Geometry check sheet. Reference: the model listing, model coordinates, mm. A direction names the side the tool comes from. Coordinates: 2 decimals unless noted, no trailing zeros. Order: outer loops, then holes, each group sorted by start corner. A loop starts at its lowest first (then second) coordinate and runs counter-clockwise, first axis right, second up. Notation, with made-up numbers: (47.25, 32) - (68.25, 32) arc R26 ccw to (68.25, 55) - close; hole circle Ø6 at (-26.75, 24). An arc over 180 degrees is marked (long way). Put each result on its own line as item: value.
Autodesk Inventor part; units mm, degrees
ref_plane "YZ Plane" through (0, 0, 0) normal (1, 0, 0) x (0, 1, 0)
ref_plane "XZ Plane" through (0, 0, 0) normal (0, 1, 0) x (-1, 0, 0)
ref_plane "XY Plane" through (0, 0, 0) normal (0, 0, 1) x (1, 0, 0)
ref_plane "Work Plane1" through (0, 0, 0) normal (0, 0, 1) x (1, 0, 0)
sketch "Sketch1" plane through (0, 0, 0) normal (0, 0, 1) x (1, 0, 0)
  circle A0 centre (-18, 0) radius 2.45 construction
  circle A1 centre (-32.0354, 0) radius 2.45 construction
  circle A2 centre (-48, 0) radius 3.05 construction
  line L0 (18, 6) -> (-54, 6) construction
  line L1 (-54, -6) -> (-54, 6) construction
  line L2 (-54, -6) -> (18, -6) construction
  line L3 (18, -6) -> (18, 6) construction
  circle A3 centre (12, 0) radius 3.05 construction
  circle A4 centre (-3.9646, 0) radius 2.45 construction
  circle A5 centre (-18, -62.5107) radius 2.45 construction
  circle A6 centre (-3.9646, -62.1646) radius 2.45 construction
  circle A7 centre (12, -70) radius 3.05 construction
  line L4 (-32.0354, -67.7344) -> (-3.9646, -67.7344) construction
  line L5 (-3.9646, -67.7344) -> (14.2856, -76.6915) construction
  line L6 (14.2856, -76.6915) -> (18.6915, -67.7144) construction
  line L7 (18.6915, -67.7144) -> (-2.5545, -57.2869) construction
  line L8 (-33.4455, -57.2869) -> (-2.5545, -57.2869) construction
  line L9 (-54.6915, -67.7144) -> (-33.4455, -57.2869) construction
  line L10 (-50.2856, -76.6915) -> (-54.6915, -67.7144) construction
  line L11 (-32.0354, -67.7344) -> (-50.2856, -76.6915) construction
  circle A8 centre (-48, -70) radius 3.05 construction
  circle A9 centre (-32.0354, -62.1646) radius 2.45 construction
  line L12 (-30, -24.7225) -> (-6, -24.7225) construction
  line L13 (-6, -24.7225) -> (-6, -18.4525) construction
  line L14 (-6, -18.4525) -> (-30, -18.4525) construction
  line L15 (-30, -18.4525) -> (-30, -24.7225) construction
  line L16 (-6, -33.7225) -> (-11.7463, -33.7225) construction
  line L17 (-6, -33.34) -> (-6, -33.7225) construction
  line L18 (-6, -33.34) -> (-11.7042, -33.34) construction
  line L19 (-6, -32.95) -> (-6, -33.34) construction
  line L20 (-6, -32.95) -> (-11.6853, -32.95) construction
  line L21 (-6, -32.56) -> (-6, -32.95) construction
  line L22 (-6, -32.56) -> (-11.6906, -32.56) construction
  line L23 (-6, -32.17) -> (-6, -32.56) construction
  line L24 (-6, -32.17) -> (-11.72, -32.17) construction
  line L25 (-6, -31.78) -> (-6, -32.17) construction
  line L26 (-6, -31.78) -> (-11.7739, -31.78) construction
  line L27 (-6, -31.39) -> (-6, -31.78) construction
  line L28 (-6, -31.39) -> (-11.8531, -31.39) construction
  line L29 (-6, -31) -> (-6, -31.39) construction
  line L30 (-6, -31) -> (-11.9583, -31) construction
  line L31 (-6, -30.61) -> (-6, -31) construction
  line L32 (-6, -30.61) -> (-12.0912, -30.61) construction
  line L33 (-6, -30.22) -> (-6, -30.61) construction
  line L34 (-6, -30.22) -> (-12.2534, -30.22) construction
  line L35 (-6, -29.83) -> (-6, -30.22) construction
  line L36 (-6, -29.83) -> (-12.4478, -29.83) construction
  line L37 (-6, -29.44) -> (-6, -29.83) construction
  line L38 (-6, -29.44) -> (-12.6777, -29.44) construction
  line L39 (-6, -29.05) -> (-6, -29.44) construction
  line L40 (-6, -29.05) -> (-12.948, -29.05) construction
  line L41 (-6, -28.66) -> (-6, -29.05) construction
  line L42 (-6, -28.66) -> (-13.2656, -28.66) construction
  line L43 (-6, -24.7225) -> (-6, -28.66) construction
  line L44 (-30, -24.7225) -> (-6, -24.7225) construction
  line L45 (-30, -28.66) -> (-30, -24.7225) construction
  line L46 (-22.7344, -28.66) -> (-30, -28.66) construction
  line L47 (-30, -29.05) -> (-30, -28.66) construction
  line L48 (-23.052, -29.05) -> (-30, -29.05) construction
  line L49 (-30, -29.44) -> (-30, -29.05) construction
  line L50 (-23.3223, -29.44) -> (-30, -29.44) construction
  line L51 (-30, -29.83) -> (-30, -29.44) construction
  line L52 (-23.5522, -29.83) -> (-30, -29.83) construction
  line L53 (-30, -30.22) -> (-30, -29.83) construction
  line L54 (-23.7466, -30.22) -> (-30, -30.22) construction
  line L55 (-30, -30.61) -> (-30, -30.22) construction
  line L56 (-23.9088, -30.61) -> (-30, -30.61) construction
  line L57 (-30, -31) -> (-30, -30.61) construction
  line L58 (-24.0417, -31) -> (-30, -31) construction
  line L59 (-30, -31.39) -> (-30, -31) construction
  line L60 (-24.1469, -31.39) -> (-30, -31.39) construction
  line L61 (-30, -31.78) -> (-30, -31.39) construction
  line L62 (-24.2261, -31.78) -> (-30, -31.78) construction
  line L63 (-30, -32.17) -> (-30, -31.78) construction
  line L64 (-24.28, -32.17) -> (-30, -32.17) construction
  line L65 (-30, -32.56) -> (-30, -32.17) construction
  line L66 (-24.3094, -32.56) -> (-30, -32.56) construction
  line L67 (-30, -32.95) -> (-30, -32.56) construction
  line L68 (-24.3147, -32.95) -> (-30, -32.95) construction
  line L69 (-30, -33.34) -> (-30, -32.95) construction
  line L70 (-24.2958, -33.34) -> (-30, -33.34) construction
  line L71 (-30, -33.7225) -> (-30, -33.34) construction
  line L72 (-24.2537, -33.7225) -> (-30, -33.7225) construction
  line L73 (-7.4129, -57.0165) -> (-7.4129, -24.5897) construction
  line L74 (-21.9151, -37.7958) -> (-30, -37.7958) construction
  line L75 (-30, -37.7958) -> (-30, -44.4525) construction
  line L76 (-30, -44.4525) -> (-6, -44.4525) construction
  line L77 (-6, -44.4525) -> (-6, -37.7958) construction
  line L78 (-6, -37.7958) -> (-14.0849, -37.7958) construction
  line L79 (-29, -9.8284) -> (-29, -53.5585)
  line L80 (-7, -53.5585) -> (-7, -9.8284)
  line L81 (-7.4685, -54.8448) -> (-16.4685, -65.5601)
  line L82 (-19.5315, -65.5601) -> (-28.5315, -54.8448)
  line L83 (-6.4142, -8.4142) -> (2, 0)
  line L84 (-7, -9) -> (4.8995, -9) construction
  line L85 (2.5858, 1.4142) -> (2.5858, 4)
  line L86 (-29.5858, -8.4142) -> (-38, 0)
  line L87 (-29, -9) -> (-17.1005, -9) construction
  line L88 (-38.5858, 1.4142) -> (-38.5858, 4)
  line L89 (0.5858, 6) -> (-36.5858, 6)
  circle A10 centre (-3.9646, 0) radius 1.45
  circle A11 centre (-32.0354, 0) radius 1.45
  circle A12 centre (-18, -62.5107) radius 1.45
  arc A13 (-19.5315, -65.5601) -> (-16.4685, -65.5601) centre (-18, -64.2738) ccw
  arc A14 (-7.4685, -54.8448) -> (-7, -53.5585) centre (-9, -53.5585) ccw
  arc A15 (-29, -53.5585) -> (-28.5315, -54.8448) centre (-27, -53.5585) ccw
  arc A16 (-6.4142, -8.4142) -> (-7, -9.8284) centre (-5, -9.8284) ccw
  arc A17 (-29, -9.8284) -> (-29.5858, -8.4142) centre (-31, -9.8284) ccw
  arc A18 (-36.5858, 6) -> (-38.5858, 4) centre (-36.5858, 4) ccw
  arc A19 (2.5858, 4) -> (0.5858, 6) centre (0.5858, 4) ccw
  arc A20 (2, 0) -> (2.5858, 1.4142) centre (0.5858, 1.4142) ccw
  arc A21 (-38.5858, 1.4142) -> (-38, 0) centre (-36.5858, 1.4142) ccw
  arc A22 (-21.9151, -37.7958) -> (-14.0849, -37.7958) centre (-18, -32.8401) ccw
  arc A23 (-24.2537, -33.7225) -> (-11.7463, -33.7225) centre (-18, -32.8401) ccw
  point P0 (0, 0)
  point P1 (2.5858, 6)
  point P2 (-38.5858, 6)
  dimension "d0" = 1
  dimension "d1" = 1
  dimension "d4" = 45
  dimension "d5" = 135
  dimension "d6" = 2.9
  dimension "d7" = 2.9
  dimension "d8" = 2.9
  dimension "d9" = 2
extrude "Extrusion1" add sketch "Sketch1" along normal blind 4
sketch "Sketch2" plane through (-29, -53.5585, 0) normal (-1, 0, 0) x (0, 0, 1)
  line L0 (-1.5567, 7.7184) -> (-1.5567, 33.7184)
  line L1 (4.4433, 27.7184) -> (4.4433, 13.7184)
  line L2 (-41.5567, 33.7184) -> (-41.5567, 7.7184)
  line L3 (10.4433, 9.1059) -> (10.4433, 35.1059)
  line L4 (10.6133, 9.1059) -> (10.6133, 15.7626)
  line L5 (4.3679, 25.1128) -> (4.3679, 21.8128)
  line L6 (4.3679, 15.0628) -> (4.3679, -1.8872)
  line L7 (3.3679, 25.1128) -> (4.3679, 25.1128)
  line L8 (3.3679, -1.8872) -> (4.3679, -1.8872)
  line L9 (5.9789, -2.5856) -> (3.3679, -2.5856)
  line L10 (3.3679, -2.5856) -> (3.3679, 27.9738)
  line L11 (3.3679, 27.9738) -> (5.9789, 27.9738)
  line L12 (5.9789, 27.9738) -> (5.9789, -2.5856)
  point P0 (0, 53.5585)
extrude "Extrusion2" cut sketch "Sketch2" against normal through all
sketch "Sketch3" plane through (-29, -44.6525, 4) normal (0, 0, 1) x (1, 0, 0)
  line L0 (0, 19.0679) -> (22, 19.0679)
  line L1 (0.4269, -10.7931) -> (24.1869, -10.7931)
  line L2 (5.8029, 16.5283) -> (16.1971, 16.5283)
  line L3 (18.1971, 14.5283) -> (18.1971, -1.4892)
  line L4 (16.1971, -3.4892) -> (5.8029, -3.4892)
  line L5 (3.8029, -1.4892) -> (3.8029, 14.5283)
  line L6 (3.8029, 16.5283) -> (18.1971, -3.4892) construction
  line L7 (18.1971, 16.5283) -> (3.8029, -3.4892) construction
  arc A0 (5.8029, 16.5283) -> (3.8029, 14.5283) centre (5.8029, 14.5283) ccw
  arc A1 (18.1971, 14.5283) -> (16.1971, 16.5283) centre (16.1971, 14.5283) ccw
  arc A2 (16.1971, -3.4892) -> (18.1971, -1.4892) centre (16.1971, -1.4892) ccw
  arc A3 (3.8029, -1.4892) -> (5.8029, -3.4892) centre (5.8029, -1.4892) ccw
  point P0 (11, 6.5196)
  dimension "d30" = 2
extrude "Extrusion3" cut sketch "Sketch3" against normal through all
chamfer "Chamfer1" [suppressed]
ref_plane "Work Plane2" through (-36.5858, -16, 0) normal (0, 1, 0) x (1, 0, 0)
properties part number "cellSTORM_inverted_chiptray_v0"
Q1. Access from +Z, -Z, +X, -X, +Y, -Y to the whole of each face (thin tool, end or side, straight path). Record for faces 4 (the flat face through (-7, -32, 2)), 5 (the flat face through (-25.5, -41.1, 3.368)), 6 (the cylindrical face through (-29.156, -9.053, 1.972)), 7 (the flat face through (-18, -48.142, 2)).
Answer block:
face 4: +Z, -Z, +X, -Y
face 5: +Z, +X, -X
face 6: +Z, -Z, -X, -Y
face 7: +Z, -Z
Q2. Section check D-D on x = -11.5. Record the boundary of the cut face in (y, z), then the cut area to 3 significant figures.
Answer block:
outline: (-59.64, 0) - (-47.66, 0) - (-47.66, 3.37) - (-56.14, 3.37) - (-56.14, 4) - (-59.64, 4) - close; (-28.61, 0) - (6, 0) - (6, 4) - (-25.58, 4) - (-25.58, 3.37) - (-28.61, 3.37) - close
area: 179 mm^2
Q3. Depth check by flat-ended pin: pin 1 Ø1.2 at (y, z) = (-42.5, 1.5) entering from -X; pin 2 Ø1.5 at (x, z) = (-33.5, 3.5) entering from -Y; pin 3 Ø1.7 at (x, y) = (-32.04, 0) entering from +Z; pin 4 Ø1 at (x, z) = (-16.5, 1.5) entering from -Y. Enter the tip coordinate at first touch or a pass-through.
Answer block:
pin 1: stops at x = -29
pin 2: stops at y = -5.25
pin 3: passes through
pin 4: stops at y = -66.01
Q4. Section check A-A on x = -18. Record the boundary of the cut face in (y, z), then the cut area to 3 significant figures.
Answer block:
outline: (-66.27, 0) - (-63.96, 0) - (-63.96, 4) - (-66.27, 4) - close; (-61.06, 0) - (-48.14, 0) - (-48.14, 3.37) - (-56.14, 3.37) - (-56.14, 4) - (-61.06, 4) - close; (-28.12, 0) - (6, 0) - (6, 4) - (-25.58, 4) - (-25.58, 3.37) - (-28.12, 3.37) - close
area: 191 mm^2
Q5. Section check C-C on z = 1.7. State how many separate pieces and enclosed holes the cut face has, then the cut area to 3 significant figures.
Answer block:
separate pieces: 1
enclosed holes: 4
area: 1,360 mm^2
Q6. Draft check along Y on faces 1 (the flat face through (-25.197, -38, 2)), 2 (the cylindrical face through (-38.015, 5.399, 1.972)), 3 (the flat face through (-2, -4, 2)). Enter one of: pulls with the +Y half, pulls with the -Y half, needs draft (parallel to the pull), parting line crosses it, or undercut.
Answer block:
face 1: undercut
face 2: pulls with the +Y half
face 3: pulls with the -Y half
Q7. Thickness scan on L1, parallel to Y at x = -18, z = 3.1; L2, parallel to X at y = -40, z = 2.3; L3, parallel to X at y = 1, z = 3.6. Record the ranges inside material, lowest first. Write a range as [from, to].
Answer block:
L1: y = [-66.27, -63.96], [-61.06, -48.14], [-28.12, 6]
L2: x = [-29, -25.2], [-10.8, -7]
L3: x = [-38.54, -33.09], [-30.99, -5.01], [-2.91, 2.54]
Q8. Section check B-B on y = -31.5. Record the boundary of the cut face in (x, z), then the cut area to 3 significant figures.
Answer block:
outline: (-29, 0) - (-25.2, 0) - (-25.2, 3.37) - (-29, 3.37) - close; (-10.8, 0) - (-7, 0) - (-7, 3.37) - (-10.8, 3.37) - close
area: 25.6 mm^2
